Can you work these out from the model? Positions are in its coordinate system, mm. A direction names the side the tool comes from. Round coordinates to 2 decimals unless told otherwise and drop trailing zeros. Order: outer loops, then holes, each group sorted by start corner. A loop starts at its lowest first (then second) coordinate and runs counter-clockwise, first axis right, second up.
Q1. If we section it at A-A (y = 37.4): Please give me the cut outline in (x, z), plus the area to 3 significant figures.
Q2. If I drill on line 1 (Y direction, x = 9, z = 10.5); line 2 (X direction, y = 62.3, z = 3.25); line 3 (Y direction, x = 24.9, z = 14.25), over which ranges is the centre line in solid material (lowest first)?
Q3. If we section it at D-D (z = 4.5): Please give me the cut outline in (x, y).
Q4. If we section it at B-B (x = 24.9): Please give me the cut outline in (y, z), plus the area to 3 significant figures.
Q5. Will these pins go through, and if not, where does the flat tip stop? P1, Ø6.5, axis at x = 29, y = 42, coming from the +Z side; P2, Ø6.5, axis at x = 9, y = 9, coming from the +Z side.
Q6. If we section it at C-C (y = 9): Please give me the cut outline in (x, z), plus the area to 3 significant figures.
Q7. We'd pull the mould along X, two halves only. Please class faces 1 (the face through (25, 71.3, 9)), 2 (the face through (0, 35, 9)), 3 (the face through (30.9, 34.9, 1.5)): pulls with the +X half, pulls with the -X half, needs draft (parallel to the pull), parting line crosses it, or undercut.
Q8. For faces 4 (the face through (30, 33, 3)), 5 (the face through (9.33, 64.83, 7.91)), which set-ups out of +Z, -Z, +X, -X, +Y, -Y let a thin tool reach every point of the face, with its end or its side?
from build123d import *

# Parameters (mm, degrees)
SKETCH1_W                       = 49.8
SKETCH1_H                       = 71.3
BASE_DEPTH                      = 18
SKETCH2_R                       = 11
LEAD_NUT_INLAY_DEPTH            = 15
SKETCH3_R                       = 6.5
LEAD_SCREW_CLEARANCE_DEPTH      = 89.253781789
WOODSCREW_CLEARANCE_D           = 5.1054
WOODSCREW_CLEARANCE_CSINK_D     = 9.779
WOODSCREW_CLEARANCE_CSINK_ANGLE = 100


with BuildPart() as part:
    # Sketch1 → base (new body)
    with BuildSketch(Plane.XY):
        with Locations((24.9, 35.65)):
            Rectangle(SKETCH1_W, SKETCH1_H)
    extrude(amount=BASE_DEPTH)

    # Sketch2 → lead nut inlay (cut)
    with BuildSketch(Plane.XY.offset(18)):
        with Locations((24.9, 37.4)):
            Circle(SKETCH2_R)
    extrude(amount=-LEAD_NUT_INLAY_DEPTH, mode=Mode.SUBTRACT)

    # Sketch3 → lead screw clearance (cut, through all)
    with BuildSketch(Plane.XY.offset(3)):
        with Locations((24.9, 37.4)):
            Circle(SKETCH3_R)
    extrude(amount=-LEAD_SCREW_CLEARANCE_DEPTH, mode=Mode.SUBTRACT)

    # woodscrew clearance (through all)
    with Locations(Plane.XY.offset(18)):
        with Locations((9, 9), (40.8, 62.3), (9, 62.3), (40.8, 9)):
            CounterSinkHole(WOODSCREW_CLEARANCE_D / 2, WOODSCREW_CLEARANCE_CSINK_D / 2, counter_sink_angle=WOODSCREW_CLEARANCE_CSINK_ANGLE)


solid = part.part
Solution:
1. outline: (0, 0) - (18.4, 0) - (18.4, 3) - (13.9, 3) - (13.9, 18) - (0, 18) - close; (31.4, 0) - (49.8, 0) - (49.8, 18) - (35.9, 18) - (35.9, 3) - (31.4, 3) - close
1. area: 527 mm2
2. line 1: y = 0 to 6.45, 11.55 to 59.75, 64.85 to 71.3
2. line 2: x = 0 to 6.45, 11.55 to 38.25, 43.35 to 49.8
2. line 3: y = 0 to 26.4, 48.4 to 71.3
3. outline: (0, 0) - (49.8, 0) - (49.8, 71.3) - (0, 71.3) - close; hole circle Ø5.11 at (9, 9); hole circle Ø5.11 at (9, 62.3); hole circle Ø22 at (24.9, 37.4); hole circle Ø5.11 at (40.8, 9); hole circle Ø5.11 at (40.8, 62.3)
4. outline: (0, 0) - (30.9, 0) - (30.9, 3) - (26.4, 3) - (26.4, 18) - (0, 18) - close; (43.9, 0) - (71.3, 0) - (71.3, 18) - (48.4, 18) - (48.4, 3) - (43.9, 3) - close
4. area: 914 mm2
5. P1: stops at z = 3
5. P2: stops at z = 16.62
6. outline: (0, 0) - (6.45, 0) - (6.45, 16.04) - (4.11, 18) - (0, 18) - close; (11.55, 0) - (38.25, 0) - (38.25, 16.04) - (35.91, 18) - (13.89, 18) - (11.55, 16.04) - close; (43.35, 0) - (49.8, 0) - (49.8, 18) - (45.69, 18) - (43.35, 16.04) - close
6. area: 703 mm2
7. face 1: needs draft
7. face 2: pulls with the -X half
7. face 3: undercut
8. face 4: +Z
8. face 5: +Z, -Z
